```python
from build123d import *

# Parameters (mm, degrees)
SKETCH1_R                      = 75
BOSS_EXTRUDE1_DEPTH            = 6.35
CBORE_FOR_M3_SHCS1_D           = 3.3
CBORE_FOR_M3_SHCS1_CBORE_D     = 6
CBORE_FOR_M3_SHCS1_CBORE_DEPTH = 3


with BuildPart() as part:
    # Sketch1 → Boss-Extrude1 (new body)
    with BuildSketch(Plane(origin=(0, 0, 0), x_dir=(1, 0, 0), z_dir=(0, 1, 0))):
        Polygon((125, 0), (88.388347648, 88.388347648), (0, 125), (-106.066017178, 106.066017178), (-198.997487421, 20), (-198.997487421, 0), (-125, 0), (-88.388347648, -88.388347648), (0, -125), (106.066017178, -106.066017178), (198.997487421, -20), (198.997487421, 0), align=None)
        with Locations(Location((0, 0, 0), (0, 0, 270))):
            Circle(SKETCH1_R, mode=Mode.SUBTRACT)
    extrude(amount=BOSS_EXTRUDE1_DEPTH)

    # CBORE for M3 SHCS1 (through all)
    with Locations(Plane.XZ):
        with Locations((90, 0), (77.942286341, 45), (45, 77.942286341), (0, 90), (-45, 77.942286341), (-77.942286341, 45), (-90, 0), (-77.942286341, -45), (-45, -77.942286341), (0, -90), (45, -77.942286341), (77.942286341, -45), (0, 0)):
            CounterBoreHole(CBORE_FOR_M3_SHCS1_D / 2, CBORE_FOR_M3_SHCS1_CBORE_D / 2, CBORE_FOR_M3_SHCS1_CBORE_DEPTH)


solid = part.part
```
Design review of the part built by this model. Coordinates are the model's own, in mm. Round coordinates to 2 decimals unless told otherwise and drop trailing zeros. Order: outer loops, then holes, each group sorted by start corner. A loop starts at its lowest first (then second) coordinate and runs counter-clockwise, first axis right, second up. Notation, with made-up numbers: M -5.5,12.25 L 35.5,12.25 A34 ccw 35.5,46.25 Z; hole C -2,-11 d7. An arc over 180 degrees is marked long. Put each result on its own line as item: value.
Q1. Consider section D-D (x = 158). State the section outline as (y, z) points, and give its area (3 significant figures).
Reported:
outline: M 0,0 L 6.35,0 L 6.35,57.97 L 0,57.97 Z
area: 368 mm²
Q2. Consider section B-B (z = -30). State the section outline as (x, y) points.
Reported:
outline: M -188.2,0 L -68.74,0 L -68.74,6.35 L -188.2,6.35 Z; M 68.74,0 L 112.57,0 L 112.57,6.35 L 68.74,6.35 Z
Q3. Consider section C-C (y = 2). State how many separate pieces and enclosed holes the cut face has, and give its area (3 significant figures).
Reported:
separate pieces: 1
enclosed holes: 13
area: 40,300 mm²
Q4. Consider section A-A (x = 29). State the section outline as (y, z) points.
Reported:
outline: M 0,-112.99 L 6.35,-112.99 L 6.35,-69.17 L 0,-69.17 Z; M 0,69.17 L 6.35,69.17 L 6.35,119.82 L 0,119.82 Z
Q5. Insertion check: pin 1 Ø2 at (x, z) = (88.5, 2) entering from -Y; pin 2 Ø2.5 at (x, z) = (-45, 77.94) entering from -Y; pin 3 Ø5 at (x, z) = (-45, -77.94) entering from -Y; pin 4 Ø3 at (x, y) = (29.5, 3) entering from +Z. Each pin has a flat end and moves straight along its axis. Give the tip position at first contact, or say it passes through.
Reported:
pin 1: y = 0
pin 2: through
pin 3: y = 3
pin 4: z = 120
Q6. To check wall thickness, follow line 1 (Z direction, x = 27, y = 6); line 2 (X direction, y = 0.5, z = -25); line 3 (X direction, y = 4, z = 16). State the ranges of each line that lie inside material, in increasing order.
Reported:
line 1: -113.82 to -69.97, 69.97 to 120.18
line 2: -193.6 to -70.71, 70.71 to 114.64
line 3: -118.37 to -73.27, 73.27 to 199
Q7. Draft analysis for pull direction Z (two halves, no side actions). For faces 1 (the face through (-3, 0, 82)), 2 (the face through (106.95, 3.13, -43.58)), 3 (the face through (-45.636, 3.131, -59.517)), 4 (the face through (-44.81, 3.13, 106.44)), state which applies: released by +Z, released by -Z, zero draft, split by the parting line, or undercut.
Reported:
face 1: zero draft
face 2: released by -Z
face 3: undercut
face 4: released by +Z
